from build123d import *

# Parameters (mm, degrees)
SKETCH2_R           = 2.5
BOSS_EXTRUDE1_DEPTH = 5


with BuildPart() as part:
    # Sketch2 → Boss-Extrude1 (new body)
    with BuildSketch(Plane.XY):
        Polygon((-31.414213562, 42.727922061), (3.313708499, 8), (106.242640687, 8), (106.242640687, -15), (-6.213203436, -15), (-47.67766953, 26.464466094), (-77.67766953, 26.464466094), (-77.67766953, 42.727922061), align=None)
        with Locations((-72.67766953, 34.596194078)):
            Circle(SKETCH2_R, mode=Mode.SUBTRACT)
        with Locations((-52.67766953, 34.596194078)):
            Circle(SKETCH2_R, mode=Mode.SUBTRACT)
        with BuildLine():
            Line((-27.878679656, 32.121320344), (-5.828427125, 10.071067812))
            ThreePointArc((-5.828427125, 10.071067812), (2.003845362, 4.83771065), (11.242640687, 3))
            Line((11.242640687, 3), (101.242640687, 3))
            Line((101.242640687, 3), (101.242640687, 0))
            Line((101.242640687, 0), (11.242640687, 0))
            ThreePointArc((11.242640687, 0), (0.855795065, 2.066072052), (-7.949747468, 7.949747468))
            Line((-7.949747468, 7.949747468), (-30, 30))
            Line((-30, 30), (-27.878679656, 32.121320344))
        make_face(mode=Mode.SUBTRACT)
        with BuildLine():
            Line((-34.949747468, 25.050252532), (-12.899494937, 3))
            ThreePointArc((-12.899494937, 3), (-1.822988962, -4.401084675), (11.242640687, -7))
            Line((11.242640687, -7), (101.242640687, -7))
            Line((101.242640687, -7), (101.242640687, -10))
            Line((101.242640687, -10), (11.242640687, -10))
            ThreePointArc((11.242640687, -10), (-2.971039259, -7.172723273), (-15.02081528, 0.878679656))
            Line((-15.02081528, 0.878679656), (-37.071067812, 22.928932188))
            Line((-37.071067812, 22.928932188), (-34.949747468, 25.050252532))
        make_face(mode=Mode.SUBTRACT)
    extrude(amount=BOSS_EXTRUDE1_DEPTH)


solid = part.part
Part model, mm, in its own coordinate system. A direction names the side the tool comes from. Round coordinates to 2 decimals unless told otherwise and drop trailing zeros. Loops run counter-clockwise (first coordinate to the right, second up) from the corner with the lowest first, then second, coordinate; pieces in that order, holes last. Notation, with made-up numbers: (-5, -29.5) - (15, -29.5) arc R25 cw to (15, 8.5) - close; hole circle Ø5 at (-26.5, -23.5). An arc over 180 degrees is marked (long way). Answer as a JSON object with one key per item and string values.
Item 1: Band-saw the part on B-B on z = 0.8. List the corners of the cut face in (x, y), plus the area to 3 significant figures.
Output:
{"outline": "(-77.68, 26.46) - (-47.68, 26.46) - (-6.21, -15) - (106.24, -15) - (106.24, 8) - (3.31, 8) - (-31.41, 42.73) - (-77.68, 42.73) - close; hole circle Ø5 at (-72.68, 34.6); hole circle Ø5 at (-52.68, 34.6); hole (-37.07, 22.93) - (-15.02, 0.88) arc R37.14 ccw to (11.24, -10) - (101.24, -10) - (101.24, -7) - (11.24, -7) arc R34.14 cw to (-12.9, 3) - (-34.95, 25.05) - close; hole (-30, 30) - (-7.95, 7.95) arc R27.14 ccw to (11.24, 0) - (101.24, 0) - (101.24, 3) - (11.24, 3) arc R24.14 cw to (-5.83, 10.07) - (-27.88, 32.12) - close", "area": "3,430 mm2"}
Item 2: Pin check, flat tips, straight feed: pin 1 (8 mm diameter, centred on x = -40.5, y = 11, fed in from +Z); pin 2 (2.5 mm diameter, centred on x = 63.5, z = 3.5, fed in from +Y); pin 3 (2 mm diameter, centred on x = -14, z = 4.5, fed in from -Y); pin 4 (1 mm diameter, centred on x = -51.5, z = 2.5, fed in from -Y). Stop position of each tip, or through.
Output:
{"pin 1": "through", "pin 2": "y = 8", "pin 3": "y = -8.21", "pin 4": "y = 26.46"}
Item 3: Band-saw the part on A-A on x = 64.5. List the corners of the cut face in (y, z), plus the area to 3 significant figures.
Output:
{"outline": "(-15, 0) - (-10, 0) - (-10, 5) - (-15, 5) - close; (-7, 0) - (0, 0) - (0, 5) - (-7, 5) - close; (3, 0) - (8, 0) - (8, 5) - (3, 5) - close", "area": "85.0 mm2"}
Item 4: Pull direction Y, two halves, no side cores. Call faces 1 (the face through (-62, 26.464, 2)), 2 (the face through (101.243, 2, 2)), 3 (the face through (14.7, 7.6, 5)): pulls with the +Y half, pulls with the -Y half, needs draft (parallel to the pull), parting line crosses it, or undercut.
Output:
{"face 1": "pulls with the -Y half", "face 2": "undercut", "face 3": "needs draft"}
Item 5: Band-saw the part on C-C on y = -5. List the corners of the cut face in (x, z), plus the area to 3 significant figures.
Output:
{"outline": "(-16.21, 0) - (-7.37, 0) - (-7.37, 5) - (-16.21, 5) - close; (-0.27, 0) - (106.24, 0) - (106.24, 5) - (-0.27, 5) - close", "area": "577 mm2"}
Item 6: Wall check: L1, parallel to Y at x = 20, z = 3.9; L2, parallel to X at y = 21.5, z = 3.55; L3, parallel to X at y = 15, z = 3.9. Give the ranges that are in metal, low to high.
Output:
{"L1": "-15 to -10, -7 to 0, 3 to 8", "L2": "-42.71 to -35.64, -31.4 to -21.5, -17.26 to -10.19", "L3": "-36.21 to -29.14, -24.9 to -15, -10.76 to -3.69"}
Item 7: Band-saw the part on D-D on y = 13. List the corners of the cut face in (x, z), plus the area to 3 significant figures.
Output:
{"outline": "(-34.21, 0) - (-27.14, 0) - (-27.14, 5) - (-34.21, 5) - close; (-22.9, 0) - (-13, 0) - (-13, 5) - (-22.9, 5) - close; (-8.76, 0) - (-1.69, 0) - (-1.69, 5) - (-8.76, 5) - close", "area": "120 mm2"}
Item 8: Tool access for faces 4 (the face through (-24.1, 14.2, 2.5)), 5 (the face through (-14.293, 25.607, 2.465)): list every direction of +Z, -Z, +X, -X, +Y, -Y with a clear straight run to the whole face (end or side of a thin tool).
Output:
{"face 4": "+Z, -Z", "face 5": "+Z, -Z, +X, +Y"}
